from build123d import *

# Parameters (mm, degrees)
SKETCH1_W                 = 31
SKETCH1_H                 = 22
BOSS_EXTRUDE1_DEPTH       = 11
SKETCH2_W                 = 31
SKETCH2_H                 = 22
SKETCH2_R                 = 7.843750423
BOSS_EXTRUDE2_DEPTH       = 5
SKETCH3_W                 = 24.5
SKETCH3_H                 = 15.5
CUT_EXTRUDE1_DEPTH        = 7.75
FILLET1_R                 = 7.75
CUT_EXTRUDE2_DEPTH        = 32.812929761
CUT_EXTRUDE2_DEPTH_BACK   = 32.812929761
SKETCH4_R                 = 5
SKETCH5_W                 = 8
SKETCH5_H                 = 8
SKETCH5_R                 = 1.905800151
BOSS_EXTRUDE3_DEPTH       = 6
CUT_EXTRUDE3_START        = -3
SKETCH6_R                 = 3
SKETCH6_R_2               = 1.905800151
CUT_EXTRUDE3_DEPTH        = 3
MIRROR9_COPY_1_SKETCH_W   = 8
MIRROR9_COPY_1_SKETCH_H   = 8
MIRROR9_COPY_1_SKETCH_R   = 1.905800151
MIRROR9_COPY_1_DEPTH      = 6
MIRROR9_START             = -3
MIRROR9_COPY_2_SKETCH_R   = 3
MIRROR9_COPY_2_SKETCH_R_2 = 1.905800151
MIRROR9_COPY_2_DEPTH      = 3
CHAMFER2_SIZE             = 4


with BuildPart() as part:
    # Sketch1 → Boss-Extrude1 (new body)
    with BuildSketch(Plane(origin=(0, 0, 0), x_dir=(1, 0, 0), z_dir=(0, 1, 0))):
        Rectangle(SKETCH1_W, SKETCH1_H)
    extrude(amount=BOSS_EXTRUDE1_DEPTH)

    # Sketch2 → Boss-Extrude2 (add)
    with BuildSketch(Plane(origin=(0, 0, 0), x_dir=(1, 0, 0), z_dir=(0, 1, 0))):
        Rectangle(SKETCH2_W, SKETCH2_H)
        with Locations(Location((0, 0, 0), (0, 0, 270))):
            Circle(SKETCH2_R, mode=Mode.SUBTRACT)
    extrude(amount=-BOSS_EXTRUDE2_DEPTH)

    # Sketch3 → Cut-Extrude1 (cut)
    with BuildSketch(Plane(origin=(0, 11, 0), x_dir=(1, 0, 0), z_dir=(0, 1, 0))):
        Rectangle(SKETCH3_W, SKETCH3_H)
    extrude(amount=-CUT_EXTRUDE1_DEPTH, mode=Mode.SUBTRACT)

    # Fillet1
    fillet1_edges = [part.edges().sort_by_distance(p)[0] for p in [
        (0, 3.25, 7.75),
        (0, 3.25, -7.75),
    ]]
    fillet(fillet1_edges, radius=FILLET1_R - 0.0001)  # a hair under: the kernel refuses the full size

    # Sketch4 → Cut-Extrude2 (cut, two sides: drawn at the far end of the back side and taken through both)
    with BuildSketch(Plane(origin=(-12.25, 0, 0), x_dir=(0, 0, -1), z_dir=(1, 0, 0)).offset(-CUT_EXTRUDE2_DEPTH_BACK)):
        with Locations((0, 11)):
            Circle(SKETCH4_R)
    extrude(amount=CUT_EXTRUDE2_DEPTH + CUT_EXTRUDE2_DEPTH_BACK, mode=Mode.SUBTRACT)

    # Sketch5 → Boss-Extrude3 (add)
    with BuildSketch(Plane(origin=(0, 11, 0), x_dir=(1, 0, 0), z_dir=(0, 1, 0))):
        with Locations((11.5, -15)):
            Rectangle(SKETCH5_W, SKETCH5_H)
        with Locations(Location((11.5, -15, 0), (0, 0, 270))):
            Circle(SKETCH5_R, mode=Mode.SUBTRACT)
    boss_extrude3 = extrude(amount=-BOSS_EXTRUDE3_DEPTH)

    # Sketch6 → Cut-Extrude3 (cut)
    with BuildSketch(Plane.XZ.offset(-5).offset(CUT_EXTRUDE3_START)):
        with Locations(Location((11.5, 15, 0), (0, 0, 270))):
            Circle(SKETCH6_R)
        with Locations(Location((11.5, 15, 0), (0, 0, 90))):
            Circle(SKETCH6_R_2, mode=Mode.SUBTRACT)
    cut_extrude3 = extrude(amount=CUT_EXTRUDE3_DEPTH, mode=Mode.SUBTRACT)

    # Mirror8: Boss-Extrude3, Cut-Extrude3 across plane
    add(boss_extrude3.mirror(Plane(origin=(0, 0, 0), x_dir=(0, 0, 1), z_dir=(1, 0, 0))))
    add(cut_extrude3.mirror(Plane(origin=(0, 0, 0), x_dir=(0, 0, 1), z_dir=(1, 0, 0))), mode=Mode.SUBTRACT)

    # Mirror9: Boss-Extrude3, Cut-Extrude3 across plane
    add(boss_extrude3.mirror(Plane.XY))
    add(cut_extrude3.mirror(Plane.XY), mode=Mode.SUBTRACT)

    # Mirror9 copy 1 sketch → Mirror9 copy 1 (add)
    with BuildSketch(Plane(origin=(0, 11, 0), x_dir=(-1, 0, 0), z_dir=(0, 1, 0))):
        with Locations((11.5, -15)):
            Rectangle(MIRROR9_COPY_1_SKETCH_W, MIRROR9_COPY_1_SKETCH_H)
        with Locations(Location((11.5, -15, 0), (0, 0, 270))):
            Circle(MIRROR9_COPY_1_SKETCH_R, mode=Mode.SUBTRACT)
    extrude(amount=-MIRROR9_COPY_1_DEPTH)

    # Mirror9 copy 2 sketch → Mirror9 copy 2 (cut)
    with BuildSketch(Plane(origin=(0, 5, 0), x_dir=(-1, 0, 0), z_dir=(0, -1, 0)).offset(MIRROR9_START)):
        with Locations(Location((11.5, 15, 0), (0, 0, 270))):
            Circle(MIRROR9_COPY_2_SKETCH_R)
        with Locations(Location((11.5, 15, 0), (0, 0, 90))):
            Circle(MIRROR9_COPY_2_SKETCH_R_2, mode=Mode.SUBTRACT)
    extrude(amount=MIRROR9_COPY_2_DEPTH, mode=Mode.SUBTRACT)

    # Chamfer2
    chamfer2_edges = [part.edges().sort_by_distance(p)[0] for p in [
        (-7.5, 8, -11),
        (7.5, 8, -11),
        (7.5, 8, 11),
        (-7.5, 8, 11),
    ]]
    chamfer(chamfer2_edges, length=CHAMFER2_SIZE)


solid = part.part
CAD build for the part. Positions are in the model's coordinates, mm. A direction names the side the tool comes from. Round coordinates to 2 decimals unless told otherwise and drop trailing zeros. Loops run counter-clockwise (first coordinate to the right, second up) from the corner with the lowest first, then second, coordinate; pieces in that order, holes last. Notation, with made-up numbers: (19.25, -16.5) - (25.25, -16.5) arc R25 ccw to (25.25, -2.5) - close; hole circle Ø11 at (62, -20.75). An arc over 180 degrees is marked (long way). Put each result on its own line as item: value.
1. Wall check: line 1 (X direction, y = 6.2, z = 15); line 2 (X direction, y = -1.45, z = 0); line 3 (Z direction, x = 13.5, y = 7.5). Give the ranges that are in metal, low to high.
Geometry check:
line 1: -15.5 to -14.5, -8.5 to -7.5, 7.5 to 8.5, 14.5 to 15.5
line 2: -15.5 to -7.84, 7.84 to 15.5
line 3: -19 to -17.24, -12.76 to -3.57, 3.57 to 12.76, 17.24 to 19
2. Slice it at D-D on z = -5.5. List the corners of the cut face in (x, y), and give its area (3 significant figures).
Geometry check:
outline: (-15.5, -5) - (-5.59, -5) - (-5.59, 0) - (5.59, 0) - (5.59, -5) - (15.5, -5) - (15.5, 11) - (12.25, 11) - (12.25, 5.54) - (-12.25, 5.54) - (-12.25, 11) - (-15.5, 11) - close
area: 306 mm²
3. Slice it at A-A on x = -11.5. Give the number of separate pieces and of enclosed holes in the cut face, and give its area (3 significant figures).
Geometry check:
separate pieces: 3
enclosed holes: 0
area: 295 mm²
4. Pin check, flat tips, straight feed: P1, Ø4, axis at x = -1, y = -2.5, coming from the +Z side; P2, Ø8, axis at x = 1.5, y = 3, coming from the +Z side; P3, Ø3, axis at x = 11.5, z = 15, coming from the +Y side; P4, Ø2.5, axis at x = 12, z = -15.5, coming from the -Y side. Stop position of each tip, or through.
Geometry check:
P1: z = 11
P2: z = 12.46
P3: through
P4: y = 8
5. Slice it at B-B on y = -1.5. List the corners of the cut face in (x, z).
Geometry check:
outline: (-15.5, -11) - (15.5, -11) - (15.5, 11) - (-15.5, 11) - close; hole circle Ø15.69 at (0, 0)
6. Two-plate mould, pull along Z, no slides. Class faces 1 (the cylindrical face through (11.584, 9.521, -13.096)), 2 (the flat face through (11, 8, -19)), 3 (the flat face through (15.5, 3, 0)): released by +Z, released by -Z, zero draft, split by the parting line, or undercut.
Geometry check:
face 1: undercut
face 2: released by -Z
face 3: zero draft
7. 3-axis set-ups, long thin cutter, end or side, ignore diameter. For faces 4 (the cylindrical face through (-11.6, 6.5, -18)), 5 (the flat face through (8, 5, -14)), 6 (the flat face through (12.25, 5, 0)), 7 (the flat face through (-7.5, 8, -17)): which of +Z, -Z, +X, -X, +Y, -Y reach the whole face in a straight line?
Geometry check:
face 4: -Y
face 5: -Z, +X, -X, -Y
face 6: +Y
face 7: -Z, +Y, -Y
